```python
from build123d import *

# Parameters (mm, degrees)
F0_W     = 1219.2
F0_H     = 1219.2
F0_W_2   = 1187.45
F0_H_2   = 15.875
F1_DEPTH = 304.8


with BuildPart() as f1:
    # F0 (on Front) → F1 (new body)
    with BuildSketch(Plane.XZ):
        with Locations((-609.6, 609.6)):
            Rectangle(F0_W, F0_H)
        Polygon((-1203.325, 946.15), (-1203.325, 1203.325), (-15.875, 1203.325), (-15.875, 946.15), (-15.875, 930.275), (-15.875, 641.35), (-15.875, 625.475), (-15.875, 336.55), (-15.875, 320.675), (-15.875, 15.875), (-1203.325, 15.875), (-1203.325, 320.675), (-1203.325, 336.55), (-1203.325, 625.475), (-1203.325, 641.35), (-1203.325, 930.275), align=None, mode=Mode.SUBTRACT)
        with Locations((-609.6, 938.2125)):
            Rectangle(F0_W_2, F0_H_2)
        with Locations((-609.6, 633.4125)):
            Rectangle(F0_W_2, F0_H_2)
        with Locations((-609.6, 328.6125)):
            Rectangle(F0_W_2, F0_H_2)
    extrude(amount=F1_DEPTH)


solid = f1.part
```
Read the model definition and answer for the solid it produces. Units are mm, in the model's axes. A direction names the side the tool comes from. Coordinates: 2 decimals unless noted, no trailing zeros. Write each loop counter-clockwise with the first axis right and the second up, starting at its lowest first coordinate (ties: lowest second). Pieces come first, ordered by that corner, then holes. Notation, with made-up numbers: (75.25, 20.5) -> (80.25, 20.5) arc R12 ccw to (80.25, 43.5) -> close; hole circle Ø3 at (76, 24). An arc over 180 degrees is marked (long way). Answer as a JSON object with one key per item and string values.
Q1. The part is cut by section A-A on z = 1077.5. Give the vertices of the cut face in (x, y) (3 decimals).
The answers:
{"outline": "(-1219.2, -304.8) -> (-1203.325, -304.8) -> (-1203.325, 0) -> (-1219.2, 0) -> close; (-15.875, -304.8) -> (0, -304.8) -> (0, 0) -> (-15.875, 0) -> close"}
Q2. The part is cut by section C-C on x = -554. Give the vertices of the cut face in (y, z) (3 decimals), then the cut area to 3 significant figures.
The answers:
{"outline": "(-304.8, 0) -> (0, 0) -> (0, 15.875) -> (-304.8, 15.875) -> close; (-304.8, 320.675) -> (0, 320.675) -> (0, 336.55) -> (-304.8, 336.55) -> close; (-304.8, 625.475) -> (0, 625.475) -> (0, 641.35) -> (-304.8, 641.35) -> close; (-304.8, 930.275) -> (0, 930.275) -> (0, 946.15) -> (-304.8, 946.15) -> close; (-304.8, 1203.325) -> (0, 1203.325) -> (0, 1219.2) -> (-304.8, 1219.2) -> close", "area": "24,200 mm2"}
Q3. Consider line 1 (Z direction, x = -915.5, y = -209.5) (3 decimals); line 2 (X direction, y = -51, z = 744.5) (3 decimals). Determine where each line is inside the solid, lowest interval first. Write a range as [from, to].
The answers:
{"line 1": "z = [0, 15.875], [320.675, 336.55], [625.475, 641.35], [930.275, 946.15], [1203.325, 1219.2]", "line 2": "x = [-1219.2, -1203.325], [-15.875, 0]"}
Q4. Determine the mould class of faces 1 (the flat face through (-15.875, -150, 170)), 2 (the flat face through (0, -150, 601)) for opening direction Z: pulls with the +Z half, pulls with the -Z half, needs draft (parallel to the pull), parting line crosses it, or undercut.
The answers:
{"face 1": "undercut", "face 2": "needs draft"}
Q5. A tool of negligible diameter and unlimited length cuts with its end or side. For faces 3 (the flat face through (-1219.2, -150, 601)), 4 (the flat face through (-618, -150, 625.475)), from which of +Z, -Z, +X, -X, +Y, -Y can it reach the whole face along a straight path? Write none if from no direction.
The answers:
{"face 3": "+Z, -Z, -X, +Y, -Y", "face 4": "+Y, -Y"}
Q6. The part is cut by section B-B on y = -178. Give the vertices of the cut face in (x, z) (3 decimals).
The answers:
{"outline": "(-1219.2, 0) -> (0, 0) -> (0, 1219.2) -> (-1219.2, 1219.2) -> close; hole (-1203.325, 15.875) -> (-15.875, 15.875) -> (-15.875, 320.675) -> (-1203.325, 320.675) -> close; hole (-1203.325, 336.55) -> (-15.875, 336.55) -> (-15.875, 625.475) -> (-1203.325, 625.475) -> close; hole (-1203.325, 641.35) -> (-15.875, 641.35) -> (-15.875, 930.275) -> (-1203.325, 930.275) -> close; hole (-1203.325, 946.15) -> (-15.875, 946.15) -> (-15.875, 1203.325) -> (-1203.325, 1203.325) -> close"}
